from build123d import *

# Parameters (mm, degrees)
EXTRUDE_1_DEPTH      = 10.8
SKETCH_2_R           = 1
EXTRUDE_2_DEPTH      = 0.8
SKETCH_3_W           = 1.7
SKETCH_3_H           = 8.1
CUT_EXTRUDE_1_DEPTH  = 17.8
EXTRUDE_START        = -4.5
EXTRUDE_3_DEPTH      = 4.5
SKETCH_5_W           = 8.4
SKETCH_5_H           = 0.05
CUT_EXTRUDE_2_DEPTH  = 1
SKETCH_6_R           = 1
CUT_EXTRUDE_3_DEPTH  = 8
CUT_EXTRUDE_4_DEPTH  = 1.2
SKETCH_8_W           = 2.8
SKETCH_8_H           = 0.608363533
EXTRUDE_4_DEPTH      = 0.1
EXTRUDE_START_2      = 2.5
EXTRUDE_5_DEPTH      = 2.5
SKETCH_10_W          = 8.4
SKETCH_10_H          = 1.7
CUT_EXTRUDE_5_DEPTH  = 0.05
FILLET_1_R           = 1.4
SKETCH_11_W          = 0.05
SKETCH_11_H          = 5.83834946
SKETCH_11_H_2        = 5.828769054
CUT_EXTRUDE_8_DEPTH  = 0.05
CUT_EXTRUDE_9_DEPTH  = 4
SKETCH_13_W          = 0.5
SKETCH_13_H          = 5.54
EXTRUDE_6_DEPTH      = 1.45
FILLET_2_R           = 1
CUT_EXTRUDE_START    = -8.12
CUT_EXTRUDE_10_DEPTH = 8.12


with BuildPart() as part:
    # Эскиз1 → Бобышка-Вытянуть1 (new body)
    with BuildSketch(Plane.XY):
        Polygon((7.4, 0), (8.4, 1), (8.4, 12.6), (0, 12.6), (0, 1), (1, 0), align=None)
    extrude(amount=EXTRUDE_1_DEPTH)

    # Эскиз2 → Бобышка-Вытянуть2 (add)
    with BuildSketch(Plane(origin=(0, 0, 0), x_dir=(-1, 0, 0), z_dir=(0, 0, -1))):
        with Locations((-4.2, 10.3)):
            Circle(SKETCH_2_R)
        with Locations((-4.2, 3.9)):
            Circle(SKETCH_2_R)
    extrude(amount=EXTRUDE_2_DEPTH)

    # Эскиз3 → Вырез-Вытянуть1 (cut)
    with BuildSketch(Plane(origin=(8.4, 0, 0), x_dir=(0, 0, -1), z_dir=(1, 0, 0))):
        with Locations((-4.75, 4.05)):
            Rectangle(SKETCH_3_W, SKETCH_3_H)
    extrude(amount=-CUT_EXTRUDE_1_DEPTH, mode=Mode.SUBTRACT)

    # Эскиз4 → Бобышка-Вытянуть3 (add)
    with BuildSketch(Plane(origin=(0, 12.6, 0), x_dir=(1, 0, 0), z_dir=(0, 1, 0)).offset(EXTRUDE_START)):
        with BuildLine():
            Line((9.1, -10.8), (-0.7, -10.8))
            Line((-0.7, -10.8), (-0.7, -2.8))
            ThreePointArc((-0.7, -2.8), (-0.992893219, -2.092893219), (-1.7, -1.8))
            Line((-1.7, -1.8), (-5.9, -1.8))
            Line((-5.9, -1.8), (-5.9, 0))
            Line((-5.9, 0), (14.3, 0))
            Line((14.3, 0), (14.3, -1.8))
            Line((14.3, -1.8), (10.1, -1.8))
            ThreePointArc((10.1, -1.8), (9.392893219, -2.092893219), (9.1, -2.8))
            Line((9.1, -2.8), (9.1, -10.8))
        make_face()
    extrude(amount=EXTRUDE_3_DEPTH)

    # Эскиз5 → Вырез-Вытянуть2 (cut)
    with BuildSketch(Plane.XY.offset(10.8)):
        with Locations((4.2, 8.075)):
            Rectangle(SKETCH_5_W, SKETCH_5_H)
    extrude(amount=-CUT_EXTRUDE_2_DEPTH, mode=Mode.SUBTRACT)

    # Эскиз6 → Вырез-Вытянуть3 (cut)
    with BuildSketch(Plane.XY.offset(10.8)):
        with Locations((4.2, 4)):
            Circle(SKETCH_6_R)
    extrude(amount=-CUT_EXTRUDE_3_DEPTH, mode=Mode.SUBTRACT)

    # Эскиз7 → Вырез-Вытянуть4 (cut)
    with BuildSketch(Plane(origin=(0, 12.6, 0), x_dir=(1, 0, 0), z_dir=(0, 1, 0))):
        with BuildLine():
            Line((8.6, 0), (8.6, -7.112411136))
            ThreePointArc((8.6, -7.112411136), (8.468198052, -7.430609188), (8.15, -7.562411136))
            Line((8.15, -7.562411136), (7.983405928, -7.562411136))
            ThreePointArc((7.983405928, -7.562411136), (7.691564003, -7.454943311), (7.539115931, -7.183870205))
            Line((7.539115931, -7.183870205), (7.049736844, -4.141202068))
            ThreePointArc((7.049736844, -4.141202068), (6.710963351, -3.53881739), (6.062425739, -3.3))
            Line((6.062425739, -3.3), (2.361664993, -3.3))
            ThreePointArc((2.361664993, -3.3), (1.71573807, -3.536600753), (1.37546474, -4.13444318))
            Line((1.37546474, -4.13444318), (0.863036378, -7.186911705))
            ThreePointArc((0.863036378, -7.186911705), (0.709913379, -7.455940797), (0.419246264, -7.562411136))
            Line((0.419246264, -7.562411136), (0.25, -7.562411136))
            ThreePointArc((0.25, -7.562411136), (-0.068198052, -7.430609188), (-0.2, -7.112411136))
            Line((-0.2, -7.112411136), (-0.2, 0))
            Line((-0.2, 0), (8.6, 0))
        make_face()
        with BuildLine():
            Line((4.2, -10.8), (5.6, -10.8))
            Line((5.6, -10.8), (5.6, -5.056380156))
            ThreePointArc((5.6, -5.056380156), (5.453553391, -4.702826765), (5.1, -4.556380156))
            Line((5.1, -4.556380156), (3.3, -4.556380156))
            ThreePointArc((3.3, -4.556380156), (2.946446609, -4.702826765), (2.8, -5.056380156))
            Line((2.8, -5.056380156), (2.8, -10.8))
            Line((2.8, -10.8), (4.2, -10.8))
        make_face()
    extrude(amount=-CUT_EXTRUDE_4_DEPTH, mode=Mode.SUBTRACT)

    # Эскиз8 → Бобышка-Вытянуть4 (add)
    with BuildSketch(Plane(origin=(0, 11.4, 0), x_dir=(1, 0, 0), z_dir=(0, 1, 0))):
        with Locations((4.2, -10.495818233)):
            Rectangle(SKETCH_8_W, SKETCH_8_H)
    extrude(amount=EXTRUDE_4_DEPTH)

    # Эскиз9 → Бобышка-Вытянуть5 (add)
    with BuildSketch(Plane.XZ.offset(-8.1).offset(EXTRUDE_START_2)):
        with BuildLine():
            Line((0, 0), (0, 3.7))
            Line((0, 3.7), (-0.7, 3.7))
            Line((-0.7, 3.7), (-0.7, 2.8))
            ThreePointArc((-0.7, 2.8), (-0.992893219, 2.092893219), (-1.7, 1.8))
            Line((-1.7, 1.8), (-5.9, 1.8))
            Line((-5.9, 1.8), (-5.9, 0))
            Line((-5.9, 0), (0, 0))
        make_face()
        with BuildLine():
            Line((14.3, 0), (8.4, 0))
            Line((8.4, 0), (8.4, 3.7))
            Line((8.4, 3.7), (9.1, 3.7))
            Line((9.1, 3.7), (9.1, 2.8))
            ThreePointArc((9.1, 2.8), (9.392893219, 2.092893219), (10.1, 1.8))
            Line((10.1, 1.8), (14.3, 1.8))
            Line((14.3, 1.8), (14.3, 0))
        make_face()
    extrude(amount=-EXTRUDE_5_DEPTH)

    # Эскиз10 → Вырез-Вытянуть5 (cut)
    with BuildSketch(Plane.XZ.offset(-8.1)):
        with Locations((4.2, 4.75)):
            Rectangle(SKETCH_10_W, SKETCH_10_H)
    extrude(amount=-CUT_EXTRUDE_5_DEPTH, mode=Mode.SUBTRACT)

    # Скругление1
    fillet_1_edges = [part.edges().sort_by_distance(p)[0] for p in [
        (-5.9, 5.6, 0.9),
        (14.3, 5.6, 0.9),
        (14.3, 12.6, 0.9),
        (-5.9, 12.6, 0.9),
    ]]
    fillet(fillet_1_edges, radius=FILLET_1_R)

    # Эскиз11 → Вырез-Вытянуть8 (cut)
    with BuildSketch(Plane(origin=(0, 0, 0), x_dir=(-1, 0, 0), z_dir=(0, 0, -1))):
        with Locations((-8.375, 8.48082527)):
            Rectangle(SKETCH_11_W, SKETCH_11_H)
        with Locations((-0.025, 8.485615473)):
            Rectangle(SKETCH_11_W, SKETCH_11_H_2)
    extrude(amount=-CUT_EXTRUDE_8_DEPTH, mode=Mode.SUBTRACT)

    # Эскиз12 → Вырез-Вытянуть9 (cut)
    with BuildSketch(Plane(origin=(0, 0, 0), x_dir=(-1, 0, 0), z_dir=(0, 0, -1))):
        with BuildLine():
            Line((1.9, 9), (1.9, 10.4))
            ThreePointArc((1.9, 10.4), (3.3, 11.8), (4.7, 10.4))
            Line((4.7, 10.4), (4.7, 9))
            ThreePointArc((4.7, 9), (3.3, 7.6), (1.9, 9))
        make_face()
        with BuildLine():
            Line((-10.3, 10.4), (-10.3, 9))
            ThreePointArc((-10.3, 9), (-11.7, 7.6), (-13.1, 9))
            Line((-13.1, 9), (-13.1, 10.4))
            ThreePointArc((-13.1, 10.4), (-11.7, 11.8), (-10.3, 10.4))
        make_face()
    extrude(amount=-CUT_EXTRUDE_9_DEPTH, mode=Mode.SUBTRACT)

    # Эскиз13 → Бобышка-Вытянуть6 (add)
    with BuildSketch(Plane(origin=(0, 11.4, 0), x_dir=(1, 0, 0), z_dir=(0, 1, 0))):
        with Locations((5.47, 0.23)):
            Rectangle(SKETCH_13_W, SKETCH_13_H)
        with Locations((8.01, 0.23)):
            Rectangle(SKETCH_13_W, SKETCH_13_H)
        with Locations((2.93, 0.23)):
            Rectangle(SKETCH_13_W, SKETCH_13_H)
        with Locations((0.39, 0.23)):
            Rectangle(SKETCH_13_W, SKETCH_13_H)
    extrude(amount=EXTRUDE_6_DEPTH)

    # Скругление2
    fillet_2_edges = [part.edges().sort_by_distance(p)[0] for p in [
        (5.47, 12.85, 2.54),
        (2.93, 12.85, 2.54),
        (0.39, 12.85, 2.54),
        (8.01, 12.85, 2.54),
    ]]
    fillet(fillet_2_edges, radius=FILLET_2_R)

    # Эскиз14 → Вырез-Вытянуть10 (cut)
    with BuildSketch(Plane.ZY.offset(-0.14).offset(CUT_EXTRUDE_START)):
        with BuildLine():
            Line((-3, 12.6), (1.54, 12.6))
            ThreePointArc((1.54, 12.6), (2.070330086, 12.380330086), (2.29, 11.85))
            Line((2.29, 11.85), (2.29, 11.4))
            Line((2.29, 11.4), (-3, 11.4))
            Line((-3, 11.4), (-3, 12.6))
        make_face()
    extrude(amount=CUT_EXTRUDE_10_DEPTH, mode=Mode.SUBTRACT)


solid = part.part
Geometry: final body of the model. Coordinates: model frame, mm. A direction names the side the tool comes from. Give positions to 0.01 mm unless a question says otherwise; leave off trailing zeros. Order: outer loops, then holes, each group sorted by start corner. A loop starts at its lowest first (then second) coordinate and runs counter-clockwise, first axis right, second up. Notation, with made-up numbers: (-16.75, -13) -> (16.25, -13) arc R18 ccw to (16.25, 4) -> close; hole circle Ø4 at (-31.75, 15). An arc over 180 degrees is marked (long way). Put each result on its own line as item: value.
Q1. Section C-C, the plane z = 8.25. Return loops of the section in (x, y).
Here are the results:
outline: (-0.7, 8.1) -> (0, 8.1) -> (0, 1) -> (1, 0) -> (7.4, 0) -> (8.4, 1) -> (8.4, 8.1) -> (9.1, 8.1) -> (9.1, 12.6) -> (5.6, 12.6) -> (5.6, 11.4) -> (2.8, 11.4) -> (2.8, 12.6) -> (-0.7, 12.6) -> close; hole circle Ø2 at (4.2, 4)
Q2. Draft query along X for faces 1 (the face through (4, 8.15, 5)), 2 (the face through (4, 6, 0)), 3 (the face through (5, 9.7, -0.4)). Return one class per face: released by +X, released by -X, zero draft, split by the parting line, or undercut.
Here are the results:
face 1: undercut
face 2: zero draft
face 3: split by the parting line
Q3. Section A-A, the plane x = -3.3. Return loops of the section in (y, z), then the cut area to 3 significant figures.
Here are the results:
outline: (5.6, 0) -> (7.6, 0) -> (7.6, 1.8) -> (5.6, 1.8) -> close; (11.8, 0) -> (12.6, 0) -> (12.6, 1.8) -> (11.8, 1.8) -> close
area: 5.04 mm^2
Q4. Pin query (flat end, axial travel): pin 1 (1 mm diameter, centred on y = 10, z = 4.5, fed in from +X); pin 2 (1.2 mm diameter, centred on y = 12.5, z = 0, fed in from -X); pin 3 (8 mm diameter, centred on x = -3, z = 5, fed in from +Y). Return the tip coordinate at first contact, or that it passes through.
Here are the results:
pin 1: stops at x = 9.1
pin 2: stops at x = -5.71
pin 3: stops at y = 12.6
Q5. Material intervals for L1, parallel to Y at x = 4.2, z = 9.15; L2, parallel to Z at x = 0.5, y = 7.75; L3, parallel to Y at x = 9, z = 8.5, sorted ascending.
Here are the results:
L1: y = 0 to 3, 5 to 11.4
L2: z = 0 to 3.9, 5.6 to 10.8
L3: y = 8.1 to 12.6
Q6. Reachability of faces 4 (the face through (3.463, 4.676, 3.358)), 5 (the face through (-1.7, 9.1, 0)), 6 (the face through (11.7, 7.6, 0.9)), 7 (the face through (7.3, 12, 5.7)) from +Z, -Z, +X, -X, +Y, -Y: full face, straight path, thin tool, end or side. Return the list, or none.
Here are the results:
face 4: +Z
face 5: -Z, -X, +Y, -Y
face 6: +Z, -Z
face 7: -Z, +Y
Q7. Section D-D, the plane y = 3.5. Return loops of the section in (x, z), then the cut area to 3 significant figures.
Here are the results:
outline: (0, 0) -> (3.28, 0) -> (3.28, -0.8) -> (5.12, -0.8) -> (5.12, 0) -> (8.4, 0) -> (8.4, 3.9) -> (5.07, 3.9) -> (5.07, 2.8) -> (3.33, 2.8) -> (3.33, 3.9) -> (0, 3.9) -> close; (0, 5.6) -> (3.33, 5.6) -> (3.33, 10.8) -> (0, 10.8) -> close; (5.07, 5.6) -> (8.4, 5.6) -> (8.4, 10.8) -> (5.07, 10.8) -> close
area: 67.0 mm^2
Q8. Section B-B, the plane z = -1.75. Return loops of the section in (x, y), then the cut area to 3 significant figures.
Here are the results:
outline: (0.14, 12.6) -> (0.64, 12.6) -> (0.64, 12.85) -> (0.14, 12.85) -> close; (2.68, 12.6) -> (3.18, 12.6) -> (3.18, 12.85) -> (2.68, 12.85) -> close; (5.22, 12.6) -> (5.72, 12.6) -> (5.72, 12.85) -> (5.22, 12.85) -> close; (7.76, 12.6) -> (8.26, 12.6) -> (8.26, 12.85) -> (7.76, 12.85) -> close
area: 0.500 mm^2
